```python
from build123d import *

# Parameters (mm, degrees)
F2_R     = 3
F3_DEPTH = 3
F4_R     = 0.75
F5_DEPTH = 3.31


# Not quite as in the source:
# - a feature names something its author has since deleted; it is built from what else it names
# - the program builds the solid bodies; features that only make, move or delete a surface that nothing else refers to are left out


with BuildPart() as f3:
    # F2 (on Top) → F3 (new body)
    with BuildSketch(Plane.XY):
        with Locations((-39.4553284803, 0)):
            Circle(F2_R)
    extrude(amount=F3_DEPTH)

    # F4 (on Front) → F5 (cut, symmetric)
    with BuildSketch(Plane.XZ):
        with Locations((-39.4553284803, 1.5)):
            Circle(F4_R)
    extrude(amount=F5_DEPTH, both=True, mode=Mode.SUBTRACT)


with BuildPart() as f3_1:
    # F8: moved
    add(f3.part.moved(Location((0.033225133, 0, -0.5896431374))))


solid = f3_1.part
```
Can you work these out from the model? Positions are in its coordinate system, mm. Round coordinates to 2 decimals unless told otherwise and drop trailing zeros. Order: outer loops, then holes, each group sorted by start corner. A loop starts at its lowest first (then second) coordinate and runs counter-clockwise, first axis right, second up.
(1) If we section it at B-B (y = -0.5): Please give me the cut outline in (x, z), plus the area to 3 significant figures.
Results are:
outline: (-42.38, -0.59) - (-36.46, -0.59) - (-36.46, 2.41) - (-42.38, 2.41) - close; hole circle Ø1.5 at (-39.42, 0.91)
area: 16.0 mm2
(2) If I drill on L1, parallel to Y at x = -39.5, z = 0.1; L2, parallel to X at y = 1, z = 1.05; L3, parallel to Z at x = -39.5, y = 2, over which ranges is the centre line in solid material (lowest first)?
Results are:
L1: y = -3 to 3
L2: x = -42.25 to -40.16, -38.69 to -36.59
L3: z = -0.59 to 0.16, 1.66 to 2.41
(3) We'd pull the mould along X, two halves only. Please class faces 1 (the face through (-38.71, -0.04, 1.14)), 2 (the face through (-36.56, 0.9, 0.89)), 3 (the face through (-39, 0, 2.41)): +X half, -X half, draft (parallel to the pull), parting line (faces both ways), or undercut.
Results are:
face 1: undercut
face 2: parting line
face 3: draft
(4) If we section it at A-A (x = -40): Please give me the cut outline in (y, z).
Results are:
outline: (-2.94, -0.59) - (2.94, -0.59) - (2.94, 0.43) - (-2.94, 0.43) - close; (-2.94, 1.39) - (2.94, 1.39) - (2.94, 2.41) - (-2.94, 2.41) - close
(5) If we section it at C-C (z = 1.1): Please give me the cut outline in (x, y).
Results are:
outline: (-40.15, -2.91) - (-40.15, 2.91) arc R3 ccw to start; (-38.7, -2.91) arc R3 ccw to (-38.7, 2.91) - close
(6) If we section it at D-D (x = -39.25): Please give me the cut outline in (y, z).
Results are:
outline: (-3, -0.59) - (3, -0.59) - (3, 0.18) - (-3, 0.18) - close; (-3, 1.64) - (3, 1.64) - (3, 2.41) - (-3, 2.41) - close
